```python
from build123d import *

# Parameters (mm, degrees)
SKETCH1_W                 = 150
SKETCH1_H                 = 40.5
MAIN_BODY_DEPTH           = 81.5
F_6_32_TAPPED_HOLE2_D     = 2.7051
F_6_32_TAPPED_HOLE2_DEPTH = 5
F_6_32_TAPPED_HOLE2_TIP   = 0.81269403
SKETCH7_W                 = 23.5
SKETCH7_H                 = 30.5
BOSS_EXTRUDE1_DEPTH       = 5


with BuildPart() as part:
    # Sketch1 → main-body (new body)
    with BuildSketch(Plane(origin=(0, 0, 0), x_dir=(0, 0, -1), z_dir=(1, 0, 0))):
        with Locations((75, 20.25)):
            Rectangle(SKETCH1_W, SKETCH1_H)
    extrude(amount=MAIN_BODY_DEPTH)

    # #6-32 Tapped Hole2
    with Locations(Plane.XY):
        with Locations((4.4, 36), (15.2, 37), (75.9, 36.25), (75.9, 4.25)):
            Hole(F_6_32_TAPPED_HOLE2_D / 2, depth=F_6_32_TAPPED_HOLE2_DEPTH)
            with Locations((0, 0, -(F_6_32_TAPPED_HOLE2_DEPTH + F_6_32_TAPPED_HOLE2_TIP / 2))):  # 118° drill point
                Cone(0, F_6_32_TAPPED_HOLE2_D / 2, F_6_32_TAPPED_HOLE2_TIP, mode=Mode.SUBTRACT)

    # Sketch7 → Boss-Extrude1 (add)
    with BuildSketch(Plane.XY):
        with Locations((15, 17.5)):
            Rectangle(SKETCH7_W, SKETCH7_H)
    extrude(amount=BOSS_EXTRUDE1_DEPTH)


solid = part.part
```
The listing builds one solid part. Answer for the finished solid, in the listing's coordinates (mm). A direction names the side the tool comes from. Give positions to 0.01 mm unless a question says otherwise; leave off trailing zeros. Order: outer loops, then holes, each group sorted by start corner. A loop starts at its lowest first (then second) coordinate and runs counter-clockwise, first axis right, second up. Notation, with made-up numbers: (31.25, 75) -> (65.25, 75) arc R29 ccw to (65.25, 95) -> close; hole circle Ø8 at (22, -26.5). An arc over 180 degrees is marked (long way). Answer as CSV lines item,"result". Start each with the question number.
Q1. Given pin 1 (4 mm diameter, centred on x = 19.5, z = 3, fed in from +Y); pin 2 (4 mm diameter, centred on y = 11, z = 2.5, fed in from +X); pin 3 (5.5 mm diameter, centred on x = 17.5, z = 3, fed in from -Y), each flat-ended and moving along its own axis, determine where each tip first touches the part or whether it passes through.
Q2. Find the intervals of material crossed by L1, parallel to X at y = 36, z = -2.65; L2, parallel to X at y = 37, z = -3.3; L3, parallel to Y at x = 15, z = -3, in increasing order.
Q3. Determine the mould class of faces 5 (the flat face through (0, 21, -74)), 6 (the conical face through (75.665, 4.26, -5.672)), 7 (the flat face through (26.75, 17, 2)), 8 (the cylindrical face through (14.58, 35.8, -2.54)) for opening direction X: pulls with the +X half, pulls with the -X half, needs draft (parallel to the pull), parting line crosses it, or undercut.
Q4. A cutting plane is placed at B-B (x = 32). Determine the outline of the cut face in (y, z), then the cut area to 4 significant figures.
Q5. A cutting plane is placed at A-A (y = 8). Determine the outline of the cut face in (x, z).
Q6. Which of the six approach directions +Z, -Z, +X, -X, +Y, -Y give full straight-line access (tool end or side, diameter ignored) to faces 1 (the cylindrical face through (76.973, 35.427, -2.535)), 2 (the flat face through (15, 32.75, 2)), 3 (the flat face through (3.25, 17, 2)), 4 (the flat face through (15, 2.25, 2))?
Results found:
1,pin 1,"y = 32.75"
1,pin 2,"x = 26.75"
1,pin 3,"y = 2.25"
2,L1,"0 to 3.05, 5.75 to 14.29, 16.11 to 74.57, 77.23 to 81.5"
2,L2,"0 to 3.49, 5.31 to 13.85, 16.55 to 74.77, 77.03 to 81.5"
2,L3,"0 to 35.66, 38.34 to 40.5"
3,face 5,"pulls with the -X half"
3,face 6,"undercut"
3,face 7,"pulls with the +X half"
3,face 8,"undercut"
4,outline,"(0, -150) -> (40.5, -150) -> (40.5, 0) -> (0, 0) -> close"
4,area,"6,075 mm2"
5,outline,"(0, -150) -> (81.5, -150) -> (81.5, 0) -> (26.75, 0) -> (26.75, 5) -> (3.25, 5) -> (3.25, 0) -> (0, 0) -> close"
6,face 1,"+Z"
6,face 2,"+Z, +X, -X, +Y"
6,face 3,"+Z, -X, +Y, -Y"
6,face 4,"+Z, +X, -X, -Y"
